Part print with two shaded views. Sizes in mm from the minimum x, y, z corner. Give positions to 0.01 mm unless a question says otherwise; leave off trailing zeros. Write each loop counter-clockwise with the first axis right and the second up, starting at its lowest first coordinate (ties: lowest second). Pieces come first, ordered by that corner, then holes. Notation, with made-up numbers: (84.5, 65.5) - (130.5, 65.5) arc R11 ccw to (130.5, 70.5) - close; hole circle Ø7 at (66.25, -20). An arc over 180 degrees is marked (long way). Answer as a JSON object with one key per item and string values.
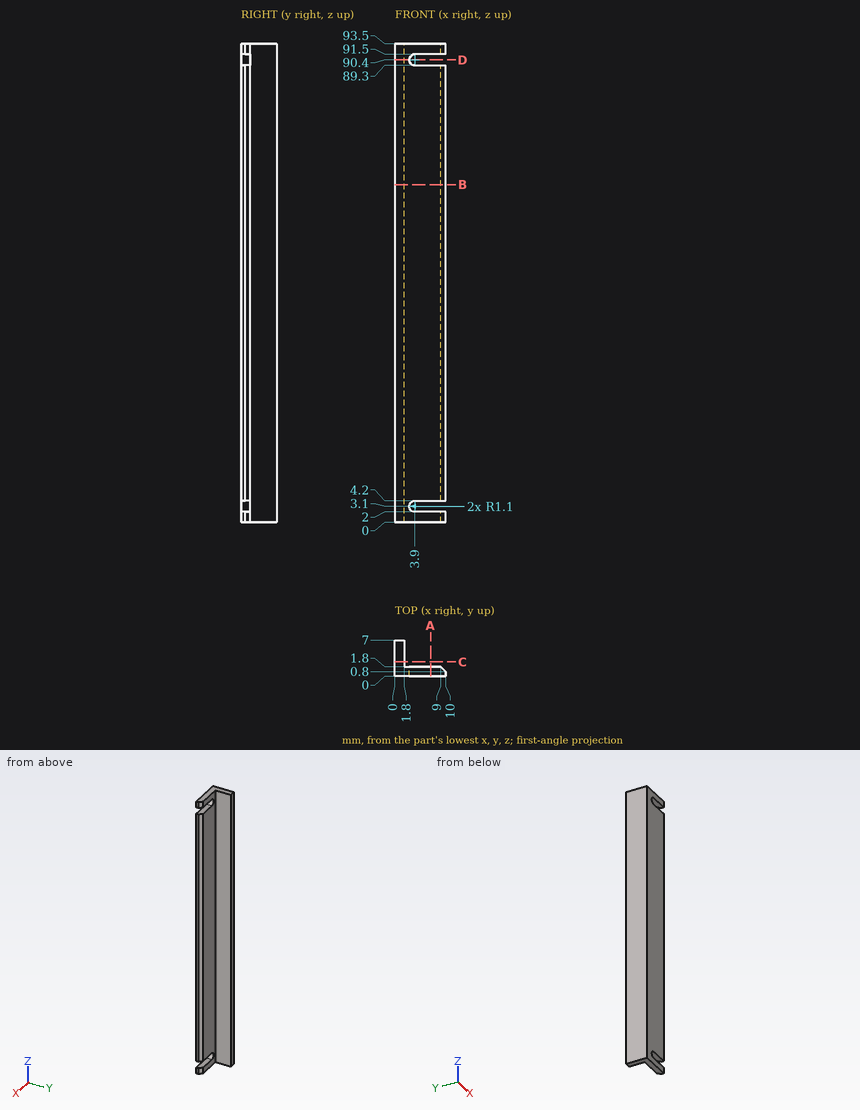
(1) Saw through at C-C, the plane y = 2.75. Give the cut face in (x, z), and give its area (3 significant figures).
Answer key:
{"outline": "(0, 0) - (1.8, 0) - (1.8, 93.5) - (0, 93.5) - close", "area": "168 mm²"}
(2) Saw through at A-A, the plane x = 7. Give the cut face in (y, z).
Answer key:
{"outline": "(0, 0) - (1.8, 0) - (1.8, 2) - (0, 2) - close; (0, 4.2) - (1.8, 4.2) - (1.8, 89.3) - (0, 89.3) - close; (0, 91.5) - (1.8, 91.5) - (1.8, 93.5) - (0, 93.5) - close"}
(3) Saw through at B-B, the plane z = 66. Give the cut face in (x, y), and give its area (3 significant figures).
Answer key:
{"outline": "(0, 0) - (10, 0) - (10, 0.8) - (9, 1.8) - (1.8, 1.8) - (1.8, 7) - (0, 7) - close", "area": "26.9 mm²"}
(4) Saw through at D-D, the plane z = 90.4. Give the cut face in (x, y), and give its area (3 significant figures).
Answer key:
{"outline": "(0, 0) - (2.8, 0) - (2.8, 1.8) - (1.8, 1.8) - (1.8, 7) - (0, 7) - close", "area": "14.4 mm²"}
(5) Probe L1, parallel to Z at x = 9.5, y = 1; L2, parallel to X at y = 5.75, z = 74. List the from-to ranges inside material, lowest first. Write a range as [from, to].
Answer key:
{"L1": "z = [0, 2], [4.2, 89.3], [91.5, 93.5]", "L2": "x = [0, 1.8]"}
(6) Flat gauge pins, fed straight in: P1, Ø1.5, axis at y = 3.5, z = 59, coming from the +X side; P2, Ø2, axis at x = 7, z = 56.5, coming from the +Y side. Where does each tip first touch, or does it go through?
Answer key:
{"P1": "stops at x = 1.8", "P2": "stops at y = 1.8"}
